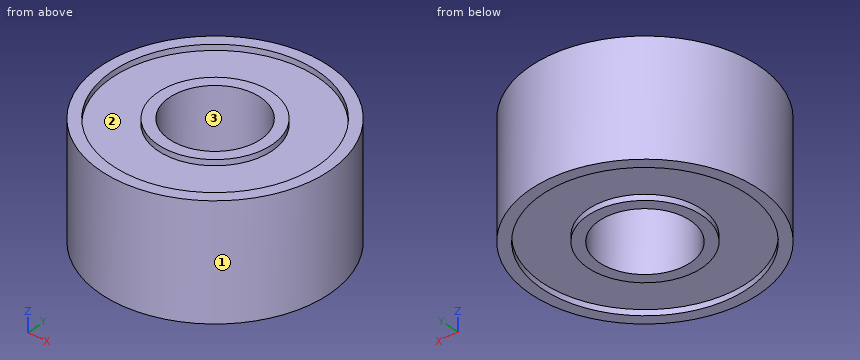
```python
from build123d import *

# Parameters (mm, degrees)
SKETCH_1_R      = 9
SKETCH_1_R_2    = 5
EXTRUDE_1_DEPTH = 4.5
SKETCH_1_3_R    = 10
SKETCH_1_3_R_2  = 9
SKETCH_1_3_R_3  = 5
SKETCH_1_3_R_4  = 4
EXTRUDE_2_DEPTH = 5


with BuildPart() as part:
    # 草图1 → 凸台-拉伸1 (new, symmetric)
    with BuildSketch(Plane.XY):
        Circle(SKETCH_1_R)
        Circle(SKETCH_1_R_2, mode=Mode.SUBTRACT)
    extrude(amount=EXTRUDE_1_DEPTH, both=True)

    # 草图1<3> → 凸台-拉伸2 (add, symmetric)
    # profile 1 of 2: a face of its own
    with BuildSketch(Plane.XY):
        Circle(SKETCH_1_3_R)
        Circle(SKETCH_1_3_R_2, mode=Mode.SUBTRACT)
    # profile 2 of 2: a face of its own
    with BuildSketch(Plane.XY):
        Circle(SKETCH_1_3_R_3)
        Circle(SKETCH_1_3_R_4, mode=Mode.SUBTRACT)
    extrude(amount=EXTRUDE_2_DEPTH, both=True)


solid = part.part
```
The listing builds one solid part. Answer for the finished solid, in the listing's coordinates (mm). Face numbers are marked on the shaded views. Round coordinates to 2 decimals unless told otherwise and drop trailing zeros. Loops run counter-clockwise (first coordinate to the right, second up) from the corner with the lowest first, then second, coordinate; pieces in that order, holes last.
Q1. Given pin 1 Ø4 at (y, z) = (-6.5, -3.5) entering from -X; pin 2 Ø6 at (x, z) = (-4, 0.5) entering from -Y; pin 3 Ø2 at (x, z) = (-1.5, 2) entering from -Y, each flat-ended and moving along its own axis, determine where each tip first touches the part or whether it passes through.
Q2. Find the intervals of material crossed by line 1 (Y direction, x = 0, z = -4.8); line 2 (Z direction, x = 6.5, y = -3); line 3 (Y direction, x = -3, z = 1.75), in increasing order.
Q3. Section A-A, the plane x = 0 is taken. Determine the outline of the cut face in (y, z), then the cut area to 3 significant figures.
Q4. Section D-D, the plane x = 6.75 is taken. Determine the outline of the cut face in (y, z).
Q5. For a pull along Y with two mould halves and no side action, classify the marked faces 1, 2 and 3 as released by +Y, released by -Y, zero draft, split by the parting line, or undercut.
Q6. Section C-C, the plane z = -3 is taken. Determine the outline of the cut face in (x, y).
Completed:
1. pin 1: stops at x = -8.93
1. pin 2: stops at y = -9.95
1. pin 3: stops at y = -9.99
2. line 1: y = -10 to -9, -5 to -4, 4 to 5, 9 to 10
2. line 2: z = -4.5 to 4.5
2. line 3: y = -9.54 to -2.65, 2.65 to 9.54
3. outline: (-10, -5) - (-9, -5) - (-9, -4.5) - (-5, -4.5) - (-5, -5) - (-4, -5) - (-4, 5) - (-5, 5) - (-5, 4.5) - (-9, 4.5) - (-9, 5) - (-10, 5) - close; (4, -5) - (5, -5) - (5, -4.5) - (9, -4.5) - (9, -5) - (10, -5) - (10, 5) - (9, 5) - (9, 4.5) - (5, 4.5) - (5, 5) - (4, 5) - close
3. area: 112 mm2
4. outline: (-7.38, -5) - (-5.95, -5) - (-5.95, -4.5) - (5.95, -4.5) - (5.95, -5) - (7.38, -5) - (7.38, 5) - (5.95, 5) - (5.95, 4.5) - (-5.95, 4.5) - (-5.95, 5) - (-7.38, 5) - close
5. face 1: split by the parting line
5. face 2: undercut
5. face 3: undercut
6. outline: circle Ø20 at (0, 0); hole circle Ø8 at (0, 0)
